from build123d import *

# Parameters (mm, degrees)
BOSS_EXTRUDE1_DEPTH = 4
CUT_EXTRUDE2_DEPTH  = 32


with BuildPart() as part:
    # Sketch1 → Boss-Extrude1 (new body)
    with BuildSketch(Plane(origin=(0, 0, 0), x_dir=(1, 0, 0), z_dir=(0, 1, 0))):
        with BuildLine():
            Line((29.180693553, -16.120036167), (29.090421484, 1.379731001))
            Line((29.090421484, 1.379731001), (29.000149416, 18.87949817))
            ThreePointArc((29.000149416, 18.87949817), (25.441707043, 27.346536312), (16.938408224, 30.817437667))
            Line((16.938408224, 30.817437667), (-18.061126113, 30.63689353))
            ThreePointArc((-18.061126113, 30.63689353), (-26.528164255, 27.078451157), (-29.99906561, 18.575152338))
            Line((-29.99906561, 18.575152338), (-29.818521473, -16.424381999))
            ThreePointArc((-29.818521473, -16.424381999), (-26.2600791, -24.891420141), (-17.756780281, -28.362321496))
            Line((-17.756780281, -28.362321496), (17.242754056, -28.181777358))
            ThreePointArc((17.242754056, -28.181777358), (25.709792198, -24.623334986), (29.180693553, -16.120036167))
        make_face()
        with BuildLine():
            ThreePointArc((17.090813971, -8.522441914), (18.840813971, -6.772441914), (17.090813971, -5.022441914))
            ThreePointArc((17.090813971, -5.022441914), (15.340813971, -6.772441914), (17.090813971, -8.522441914))
        make_face(mode=Mode.SUBTRACT)
        with BuildLine():
            ThreePointArc((-17.909186029, -5.022441914), (-19.659186029, -6.772441914), (-17.909186029, -8.522441914))
            ThreePointArc((-17.909186029, -8.522441914), (-16.159186029, -6.772441914), (-17.909186029, -5.022441914))
        make_face(mode=Mode.SUBTRACT)
        with BuildLine():
            ThreePointArc((-0.409186029, 5.727558086), (-4.909186029, 1.227558086), (-0.409186029, -3.272441914))
            ThreePointArc((-0.409186029, -3.272441914), (4.090813971, 1.227558086), (-0.409186029, 5.727558086))
        make_face(mode=Mode.SUBTRACT)
    extrude(amount=BOSS_EXTRUDE1_DEPTH)

    # Sketch2 → Cut-Extrude2 (cut)
    with BuildSketch(Plane(origin=(0, 4, 0), x_dir=(1, 0, 0), z_dir=(0, 1, 0))):
        Polygon((-24.831482976, -13.898822811), (-24.986237153, 16.101177189), (-29.98617063, 16.07538517), (-29.831416453, -13.92461483), align=None)
        Polygon((29.167798572, -13.620268999), (29.013044396, 16.379731001), (24.013110919, 16.353938982), (24.167865096, -13.646061018), align=None)
    extrude(amount=-CUT_EXTRUDE2_DEPTH, mode=Mode.SUBTRACT)


solid = part.part
Verification items for the finished model (mm, model axes). Give positions to 0.01 mm unless a question says otherwise; leave off trailing zeros. Loops run counter-clockwise (first coordinate to the right, second up) from the corner with the lowest first, then second, coordinate; pieces in that order, holes last.
1) Draft check along Z on faces 1 (the flat face through (-1, 4, 5)), 2 (the cylindrical face through (-0.211, 1.972, -5.723)), 3 (the cylindrical face through (25.535, 1.972, -27.253)), 4 (the cylindrical face through (15.356, 1.972, 7)). Enter one of: pulls with the +Z half, pulls with the -Z half, needs draft (parallel to the pull), parting line crosses it, or undercut.
2) Sectioned sample at A-A, the plane z = -3.5. Enter the section's corners in (x, y), then the cut area to 3 significant figures.
3) Thickness scan on line 1 along X through (y, z) = (2.55, -14); line 2 along Z through (x, y) = (-17.5, 3.2); line 3 along X through (y, z) = (1.4, 5.5). Record the ranges inside material, lowest first.
4) Sectioned sample at D-D, the plane z = 6.5. Enter the section's corners in (x, y), then the cut area to 3 significant figures.
5) Sectioned sample at B-B, the plane y = 2.65. Enter the section's corners in (x, z), then the cut area to 3 significant figures.
6) Depth check by flat-ended pin: pin 1 Ø1 at (x, y) = (18.5, 3) entering from +Z. Enter the tip coordinate at first touch or a pass-through.
7) Sectioned sample at C-C, the plane x = 25.5. Enter the section's corners in (y, z).
Answers:
1. face 1: needs draft
1. face 2: undercut
1. face 3: pulls with the -Z half
1. face 4: undercut
2. outline: (-24.92, 0) - (-4.29, 0) - (-4.29, 4) - (-24.92, 4) - close; (3.47, 0) - (24.08, 0) - (24.08, 4) - (3.47, 4) - close
2. area: 165 mm2
3. line 1: x = -24.98 to 24.03
3. line 2: z = -30.64 to 5.07, 8.47 to 28.36
3. line 3: x = -24.87 to -19.11, -16.71 to 15.89, 18.29 to 24.13
4. outline: (-24.87, 0) - (-19.64, 0) - (-19.64, 4) - (-24.87, 4) - close; (-16.18, 0) - (15.36, 0) - (15.36, 4) - (-16.18, 4) - close; (18.82, 0) - (24.13, 0) - (24.13, 4) - (18.82, 4) - close
4. area: 168 mm2
5. outline: (-30, -18.58) arc R12 ccw to (-18.06, -30.64) - (16.94, -30.82) arc R12 ccw to (29, -18.88) - (29.01, -16.38) - (24.01, -16.35) - (24.17, 13.65) - (29.17, 13.62) - (29.18, 16.12) arc R12 ccw to (17.24, 28.18) - (-17.76, 28.36) arc R12 ccw to (-29.82, 16.42) - (-29.83, 13.92) - (-24.83, 13.9) - (-24.99, -16.1) - (-29.99, -16.08) - close; hole circle Ø3.5 at (-17.91, 6.77); hole circle Ø9 at (-0.41, -1.23); hole circle Ø3.5 at (17.09, 6.77)
5. area: 2,970 mm2
6. pin 1: stops at z = 28.15
7. outline: (0, -27.29) - (4, -27.29) - (4, -16.36) - (0, -16.36) - close; (0, 13.64) - (4, 13.64) - (4, 24.83) - (0, 24.83) - close
